```python
from build123d import *

# Parameters (mm, degrees)
EXTRUDE1_DEPTH = 0.25
FILLET1_R      = 0.25


with BuildPart() as part:
    # Sketch1 → Revolve1 (revolve)
    with BuildSketch(Plane(origin=(0, 0, 0), x_dir=(0, 0, -1), z_dir=(1, 0, 0)), mode=Mode.PRIVATE) as revolve1_sk:
        with BuildLine():
            Line((0, 1.45), (2.15, 1.45))
            Line((2.15, 1.45), (2.15, 1.599999975))
            Line((2.15, 1.599999975), (3.15, 1.599999975))
            Line((3.15, 1.599999975), (3.15, 0))
            Line((3.15, 0), (-1.45, 0))
            ThreePointArc((-1.45, 0), (-1.025304833, 1.025304833), (0, 1.45))
        make_face()
    revolve(revolve1_sk.sketch.rotate(Axis((0, 0, 0), (0, 0, -1)), 90), axis=Axis((0, 0, 0), (0, 0, -1)))

    # Sketch2 → Extrude1 (add, symmetric)
    with BuildSketch(Plane(origin=(0, 0, 0), x_dir=(0, 0, -1), z_dir=(1, 0, 0))):
        with BuildLine():
            Line((3.15, 1.026953873), (3.95, 1.4))
            Line((3.95, 1.4), (6.15, 1.4))
            Line((6.15, 1.4), (6.15, 1.5))
            Line((6.15, 1.5), (7.15, 1.5))
            Line((7.15, 1.5), (7.15, 1.4))
            Line((7.15, 1.4), (30.15, 1.4))
            Line((30.15, 1.4), (30.15, 0.9))
            Line((30.15, 0.9), (7.15, 0.9))
            Line((7.15, 0.9), (7.15, 0.8))
            Line((7.15, 0.8), (6.15, 0.8))
            Line((6.15, 0.8), (6.15, 0.9))
            Line((6.15, 0.9), (4.05, 0.9))
            ThreePointArc((4.05, 0.9), (3.979289322, 0.870710678), (3.95, 0.8))
            Line((3.95, 0.8), (3.95, 0.5))
            Line((3.95, 0.5), (3.15, 0.5))
            Line((3.15, 0.5), (3.15, 1.026953873))
        make_face()
        with BuildLine():
            Line((3.95, -0.8), (3.95, -0.5))
            Line((3.95, -0.5), (3.15, -0.5))
            Line((3.15, -0.5), (3.15, -1.026953873))
            Line((3.15, -1.026953873), (3.95, -1.4))
            Line((3.95, -1.4), (6.15, -1.4))
            Line((6.15, -1.4), (6.15, -1.5))
            Line((6.15, -1.5), (7.15, -1.5))
            Line((7.15, -1.5), (7.15, -1.4))
            Line((7.15, -1.4), (30.15, -1.4))
            Line((30.15, -1.4), (30.15, -0.9))
            Line((30.15, -0.9), (7.15, -0.9))
            Line((7.15, -0.9), (7.15, -0.8))
            Line((7.15, -0.8), (6.15, -0.8))
            Line((6.15, -0.8), (6.15, -0.9))
            Line((6.15, -0.9), (4.05, -0.9))
            ThreePointArc((4.05, -0.9), (3.979289322, -0.870710678), (3.95, -0.8))
        make_face()
    extrude(amount=EXTRUDE1_DEPTH, both=True)

    # Fillet1
    fillet1_edges = [part.edges().sort_by_distance(p)[0] for p in [
        (-0.25, 0.763476937, -3.15),
        (0, 1.026953873, -3.15),
        (0, 0.5, -3.15),
        (0.25, 0.763476937, -3.15),
        (-0.25, -0.763476937, -3.15),
        (0, -0.5, -3.15),
        (0, -1.026953873, -3.15),
        (0.25, -0.763476937, -3.15),
    ]]
    fillet(fillet1_edges, radius=FILLET1_R)


solid = part.part
```
Model file for the job. Use its own axes, mm. A direction names the side the tool comes from. Give positions to 0.01 mm unless a question says otherwise; leave off trailing zeros. Write each loop counter-clockwise with the first axis right and the second up, starting at its lowest first coordinate (ties: lowest second). Pieces come first, ordered by that corner, then holes. Notation, with made-up numbers: M 41.25,74.5 L 65.25,74.5 A17 ccw 65.25,92.5 Z; hole C -22.75,-14 d9. An arc over 180 degrees is marked long. Use a Markdown table: item, result.
1) Drill centre lines: line 1 (X direction, y = -1.35, z = -24); line 2 (Z direction, x = -0.8, y = -0.15); line 3 (Y direction, x = -0.05, z = -5.5). Where is each one in solid material? Low to high. Write a range as from..to.
Responses:
| item | result |
|---|---|
| line 1 | x = -0.25..0.25 |
| line 2 | z = -3.15..1.2 |
| line 3 | y = -1.4..-0.9, 0.9..1.4 |
2) Tool access for faces 1 (the flat face through (-0.25, -1.1, -16.6)), 2 (the cylindrical face through (-1.45, -0.06, -1.09)), 3 (the flat face through (0.25, -1.1, -16.6)): list every direction of +Z, -Z, +X, -X, +Y, -Y with a clear straight run to the whole face (end or side of a thin tool).
Responses:
| item | result |
|---|---|
| face 1 | -Z, -X, +Y, -Y |
| face 2 | +Z |
| face 3 | -Z, +X, +Y, -Y |
3) Cut at B-B (x = -1.1). List the corners of the cut face in (y, z), and give its area (3 significant figures).
Responses:
| item | result |
|---|---|
| outline | M -1.16,-3.15 L 1.16,-3.15 L 1.16,-2.15 L 0.94,-2.15 L 0.94,0 A0.94 ccw -0.94,0 L -0.94,-2.15 L -1.16,-2.15 Z |
| area | 7.79 mm2 |
4) Cut at A-A (z = -21). List the corners of the cut face in (x, y).
Responses:
| item | result |
|---|---|
| outline | M -0.25,-1.4 L 0.25,-1.4 L 0.25,-0.9 L -0.25,-0.9 Z; M -0.25,0.9 L 0.25,0.9 L 0.25,1.4 L -0.25,1.4 Z |
5) Pin check, flat tips, straight feed: pin 1 (1 mm diameter, centred on y = 0.5, z = -19, fed in from -X); pin 2 (0.6 mm diameter, centred on x = 0, z = -7, fed in from +Y). Stop position of each tip, or through.
Responses:
| item | result |
|---|---|
| pin 1 | stops at x = -0.25 |
| pin 2 | stops at y = 1.5 |
